Check sheet for the modelled part. Datum: model origin and axes. Units: mm. A direction names the side the tool comes from. Round coordinates to 2 decimals unless told otherwise and drop trailing zeros. Loops run counter-clockwise (first coordinate to the right, second up) from the corner with the lowest first, then second, coordinate; pieces in that order, holes last. Notation, with made-up numbers: (28.25, 59.5) - (66.25, 59.5) arc R17 ccw to (66.25, 80.5) - close; hole circle Ø2 at (48.5, -15.5). An arc over 180 degrees is marked (long way). Put each result on its own line as item: value. Start each with the question number.
Item 1: Section check A-A, the plane y = 190.5. Record the cut outline in (x, z) (3 decimals), and give its area (3 significant figures).
Item 2: Gauge pin test, flat ends, axial feed: pin 1 Ø5.5 at (y, z) = (133.35, 12.7) entering from +X (3 decimals); pin 2 Ø2 at (x, z) = (-2, 20.5) entering from -Y; pin 3 Ø1.7 at (x, y) = (-3, 141) entering from +Z; pin 4 Ø3 at (y, z) = (133.35, 38.1) entering from -X. Record the tip position at first contact, or that the pin passes through.
Item 3: Tool access check on faces 5 (the cylindrical face through (-3.58, 234.92, 46.44)), 6 (the conical face through (-18.41, 232.5, 52.18)), 7 (the flat face through (-3.579, 266.315, 21.295)). Record the directions out of +Z, -Z, +X, -X, +Y, -Y that give a thin tool (end or side, any length) a straight path to the whole face; none if there is none.
Item 4: Draft check along Z on faces 1 (the conical face through (-0.132, 253.065, 1.993)), 2 (the flat face through (-8.02, 248.12, 54.8)), 3 (the conical face through (-0.56, 250.98, 7.1)), 4 (the conical face through (-0.64, 232.5, 52.18)). Enter one of: pulls with the +Z half, pulls with the -Z half, needs draft (parallel to the pull), parting line crosses it, or undercut.
Item 5: Material ranges on line 1 along Z through (x, y) = (-13.5, 63.5); line 2 along Z through (x, y) = (-14.25, 114.3) (3 decimals); line 3 along Z through (x, y) = (-3, 178), recorded low to high.
from build123d import *

# Parameters (mm, degrees)
F1_DEPTH = 19.05
F2_R     = 19.05
F4_DEPTH = 9.525
F5_SIZE  = 3.048
F6_R     = 9.525
F7_DEPTH = 9.526
F8_SIZE  = 0.762
F10_D    = 7.112
F12_D    = 3.302


with BuildPart() as f1:
    # F0 (on Right) → F1 (new body)
    with BuildSketch(Plane.YZ):
        Polygon((0, 50.8), (0, 0), (254, 0), (295.819744, 41.819744), (259.898719, 77.740768), (232.957951, 50.8), align=None)
    extrude(amount=-F1_DEPTH)

    # F2
    f2_edges = [f1.edges().sort_by_distance(p)[0] for p in [
        (-9.525, 259.898719, 77.740768),
        (-9.525, 295.819744, 41.819744),
        (-9.525, 232.957951, 50.8),
        (-9.525, 254, 0),
    ]]
    fillet(f2_edges, radius=F2_R)

    # F3 (on face) → F4 (cut)
    with BuildSketch(Plane.YZ):
        with BuildLine():
            ThreePointArc((243.027695, 51.889488), (234.787342, 46.38346), (225.067183, 44.45))
            Line((225.067183, 44.45), (0, 44.45))
            Line((0, 44.45), (0, 6.35))
            Line((0, 6.35), (246.109232, 6.35))
            ThreePointArc((246.109232, 6.35), (250.969311, 7.31673), (255.089488, 10.069744))
            Line((255.089488, 10.069744), (277.859232, 32.839488))
            ThreePointArc((277.859232, 32.839488), (281.578976, 41.819744), (277.859232, 50.8))
            Line((277.859232, 50.8), (268.878976, 59.780256))
            ThreePointArc((268.878976, 59.780256), (259.898719, 63.5), (250.918463, 59.780256))
            Line((250.918463, 59.780256), (243.027695, 51.889488))
        make_face()
    extrude(amount=-F4_DEPTH, mode=Mode.SUBTRACT)

    # F5
    f5_edges = [f1.edges().sort_by_distance(p)[0] for p in [
        (-9.525, 112.533591, 44.45),
    ]]
    chamfer(f5_edges, length=F5_SIZE)

    # F6 (on face) → F7 (cut, through all)
    with BuildSketch(Plane.YZ.offset(-9.525)):
        with Locations((76.2, 25.4)):
            Circle(F6_R)
        with Locations((114.3, 25.4)):
            Circle(F6_R)
        with Locations((152.4, 25.4)):
            Circle(F6_R)
        with Locations((259.898719, 41.819744)):
            Circle(F6_R)
        with Locations((190.5, 25.4)):
            Circle(F6_R)
        with Locations((228.014071, 25.4)):
            Circle(F6_R)
    extrude(amount=-F7_DEPTH, mode=Mode.SUBTRACT)

    # F8
    f8_edges = [f1.edges().sort_by_distance(p)[0] for p in [
        (-9.525, 66.675, 25.4),
        (-9.525, 104.775, 25.4),
        (-9.525, 142.875, 25.4),
        (-9.525, 180.975, 25.4),
        (-9.525, 218.489071, 25.4),
        (-9.525, 250.373719, 41.819744),
        (0, 123.054616, 0),
        (0, 266.47436, 21.454616),
        (-19.05, 123.054616, 0),
    ]]
    chamfer(f8_edges, length=F8_SIZE)

    # F10 (through all)
    with Locations(Plane.YZ.offset(-9.525)):
        with Locations((50.8, 25.4), (12.7, 25.4)):
            Hole(F10_D / 2)

    # F12 (through all)
    with Locations(Plane.YZ.offset(-9.525)):
        with Locations((247.65, 12.7), (240.714071, 38.1), (209.55, 12.7), (209.55, 38.1), (171.45, 12.7), (171.45, 38.1), (133.35, 12.7), (133.35, 38.1), (95.25, 12.7), (95.25, 38.1), (63.5, 12.7), (63.5, 38.1)):
            Hole(F12_D / 2)


solid = f1.part
Check result:
1. outline: (-19.05, 0.762) - (-18.288, 0) - (-0.762, 0) - (0, 0.762) - (0, 5.588) - (-0.762, 6.35) - (-6.477, 6.35) - (-9.525, 9.398) - (-9.525, 15.113) - (-10.287, 15.875) - (-19.05, 15.875) - close; (-19.05, 34.925) - (-10.287, 34.925) - (-9.525, 35.687) - (-9.525, 41.402) - (-6.477, 44.45) - (-0.762, 44.45) - (0, 45.212) - (0, 50.038) - (-0.762, 50.8) - (-18.288, 50.8) - (-19.05, 50.038) - close
1. area: 430 mm²
2. pin 1: x = -9.525
2. pin 2: y = 264.52
2. pin 3: z = 50.8
2. pin 4: through
3. face 5: +X
3. face 6: +Z, -X, -Y
3. face 7: +X, -Y
4. face 1: pulls with the -Z half
4. face 2: undercut
4. face 3: undercut
4. face 4: pulls with the +Z half
5. line 1: 0 to 11.05, 14.35 to 36.45, 39.75 to 50.8
5. line 2: 0 to 15.875, 34.925 to 50.8
5. line 3: 0 to 6.35, 44.45 to 50.8
